```python
from build123d import *

# Parameters (mm, degrees)
PAD_DEPTH    = 20.32
POCKET_DEPTH = 21


with BuildPart() as part:
    # Sketch → Pad (new body)
    with BuildSketch(Plane.XY):
        Polygon((0, 0), (0, 2.51), (5, 2.51), (4.999966, 8.51), (123.5, 8.51), (123.5, 2.51), (128.5, 2.51), (128.5, 0), align=None)
    extrude(amount=PAD_DEPTH)

    # Sketch002 → Pocket (cut)
    with BuildSketch(Plane.XZ):
        with BuildLine():
            ThreePointArc((20, 5), (15, 0), (20, -5))
            Line((20, -5), (40, -5))
            ThreePointArc((40, -5), (45, 0), (40, 5))
            Line((40, 5), (20, 5))
        make_face()
        with BuildLine():
            ThreePointArc((20, 25.32), (15, 20.32), (20, 15.32))
            Line((20, 15.32), (40, 15.32))
            ThreePointArc((40, 15.32), (45, 20.32), (40, 25.32))
            Line((40, 25.32), (20, 25.32))
        make_face()
    extrude(amount=-POCKET_DEPTH, mode=Mode.SUBTRACT)


solid = part.part
```
The model under review builds one solid part; all positions refer to its coordinate system, in mm. A direction names the side the tool comes from. Round coordinates to 2 decimals unless told otherwise and drop trailing zeros. Write each loop counter-clockwise with the first axis right and the second up, starting at its lowest first coordinate (ties: lowest second). Pieces come first, ordered by that corner, then holes. Notation, with made-up numbers: (-2.75, 50) - (13.25, 50) arc R27 ccw to (13.25, 79) - close; hole circle Ø3 at (-0.5, 85). An arc over 180 degrees is marked (long way). Answer as CSV lines item,"result". Start each with the question number.
(1) For pin 1 Ø5 at (y, z) = (6, 7.5) entering from +X; pin 2 Ø2.5 at (x, z) = (2, 6) entering from +Y; pin 3 Ø4.5 at (x, y) = (29, 4) entering from -Z, all flat-tipped, find the tip position at first contact; note any pin that passes through.
(2) Draft analysis for pull direction X (two halves, no side actions). For faces 6 (the flat face through (63, 8.51, 10)), 7 (the cylindrical face through (43.5, 4.2, 16.75)), 8 (the flat face through (123.5, 6, 10)), state which applies: pulls with the +X half, pulls with the -X half, needs draft (parallel to the pull), parting line crosses it, or undercut.
(3) We need section A-A on z = 18.5. State the section outline as (x, y) points.
(4) To check wall thickness, follow line 1 (X direction, y = 7, z = 6.25); line 2 (X direction, y = 4.75, z = 1.5); line 3 (X direction, y = 4.75, z = 2). State the ranges of each line that lie inside material, in increasing order.
(5) We need section D-D on x = 29. State the section outline as (y, z) points.
(6) For faces 1 (the flat face through (126, 2.51, 10)), 2 (the flat face through (128.5, 1, 10)), 3 (the flat face through (2, 2.51, 10)), 4 (the cylindrical face through (17, 4, 4)), 5 (the flat face through (30, 4, 15.32)), list the 3-axis set-ups (+Z, -Z, +X, -X, +Y, -Y) from which the entire face can be reached by the end or side of a thin tool; tool diameter is ignored.
(7) We need section C-C on y = 4.75. State the section outline as (x, z) points.
(8) We need section B-B on z = 13.5. State the section outline as (x, y) points.
Worked answers:
1,pin 1,"x = 123.5"
1,pin 2,"y = 2.51"
1,pin 3,"z = 5"
2,face 6,"needs draft"
2,face 7,"undercut"
2,face 8,"pulls with the +X half"
3,outline,"(0, 0) - (15.34, 0) - (15.34, 8.51) - (5, 8.51) - (5, 2.51) - (0, 2.51) - close; (44.66, 0) - (128.5, 0) - (128.5, 2.51) - (123.5, 2.51) - (123.5, 8.51) - (44.66, 8.51) - close"
4,line 1,"5 to 123.5"
4,line 2,"5 to 15.23, 44.77 to 123.5"
4,line 3,"5 to 15.42, 44.58 to 123.5"
5,outline,"(0, 5) - (8.51, 5) - (8.51, 15.32) - (0, 15.32) - close"
6,face 1,"+Z, -Z, +X, +Y"
6,face 2,"+Z, -Z, +X, +Y, -Y"
6,face 3,"+Z, -Z, -X, +Y"
6,face 4,"-Z, +Y, -Y"
6,face 5,"+Z, +Y, -Y"
7,outline,"(5, 0) - (15, 0) arc R5 cw to (20, 5) - (40, 5) arc R5 cw to (45, 0) - (123.5, 0) - (123.5, 20.32) - (45, 20.32) arc R5 cw to (40, 15.32) - (20, 15.32) arc R5 cw to (15, 20.32) - (5, 20.32) - close"
8,outline,"(0, 0) - (128.5, 0) - (128.5, 2.51) - (123.5, 2.51) - (123.5, 8.51) - (5, 8.51) - (5, 2.51) - (0, 2.51) - close"
